Design review of the part built by this model. Coordinates are the model's own, in mm. A direction names the side the tool comes from. Coordinates: 2 decimals unless noted, no trailing zeros. Loops run counter-clockwise (first coordinate to the right, second up) from the corner with the lowest first, then second, coordinate; pieces in that order, holes last. Notation, with made-up numbers: (83.5, 25.25) -> (108.5, 25.25) arc R28 ccw to (108.5, 45.25) -> close; hole circle Ø11 at (61.25, -22.5). An arc over 180 degrees is marked (long way). Answer as a JSON object with one key per item and string values.
Autodesk Inventor part; units mm, degrees
ref_plane "YZ Plane" through (0, 0, 0) normal (1, 0, 0) x (0, 1, 0)
ref_plane "XZ Plane" through (0, 0, 0) normal (0, 1, 0) x (-1, 0, 0)
ref_plane "XY Plane" through (0, 0, 0) normal (0, 0, 1) x (1, 0, 0)
sketch "Szkic1" plane through (0, 0, 0) normal (0, 1, 0) x (-1, 0, 0)
  point P0 (0, 0)
sketch "Szkic2" plane through (0, 0, 0) normal (1, 0, 0) x (0, 1, 0)
  point P0 (0, 0)
sketch "Szkic3" plane through (0, 0, 0) normal (1, 0, 0) x (0, 1, 0)
  line L0 (0, 0) -> (30, 0)
  line L1 (30, 0) -> (30, -36)
  line L2 (30, -36) -> (0, -36)
  line L3 (0, -5) -> (-3, -5)
  line L4 (-3, -5) -> (-3, -31)
  line L5 (-3, -31) -> (0, -31)
  line L6 (0, -36) -> (0, -31)
  line L7 (0, -5) -> (0, 0)
  arc A0 (14.6923, -17.4615) -> (19.3077, -17.4615) centre (17, -23) ccw
  arc A1 (19.3077, -17.4615) -> (14.6923, -17.4615) centre (17, -16.5) ccw
  circle A2 centre (17, -31.5) radius 1.25
  circle A3 centre (17, -4.5) radius 1.25
  dimension "d1" = 36
  dimension "d4" = 5
  dimension "d5" = 26
  dimension "d6" = 3
  dimension "d7" = 30
  dimension "d8" = 13
  dimension "d9" = 13
  dimension "d10" = 4.5
  dimension "d11" = 4.5
  dimension "d12" = 6.5
  dimension "d13" = 12
  dimension "d14" = 5
  dimension "d15" = 2.5
  dimension "d16" = 2.5
extrude "Wyciągnięcie proste1" add sketch "Szkic3" along normal blind 3
properties part number "Podstawa-mocowanie serwa" material "Drewno (wiśnia)"
1) Clearance check with a flat-ended pin moving along its axis: pin 1 Ø11 at (y, z) = (17, -23) entering from +X. State where the tip first meets the part, or that it passes through.
Completed:
{"pin 1": "through"}
2) Add section C-C, the plane x = 0.4. Give the boundary of the cut face in (y, z), and give its area (3 significant figures).
Completed:
{"outline": "(-3, -31) -> (0, -31) -> (0, -36) -> (30, -36) -> (30, 0) -> (0, 0) -> (0, -5) -> (-3, -5) -> close; hole (14.69, -17.46) arc R6 ccw (long way) to (19.31, -17.46) arc R2.5 ccw (long way) to start; hole circle Ø2.5 at (17, -31.5); hole circle Ø2.5 at (17, -4.5)", "area": "1,020 mm²"}
3) For faces 5 (the flat face through (1, -1, -5)), 6 (the flat face through (1, 0, -34)), 7 (the flat face through (1, 30, -18)), list the 3-axis set-ups (+Z, -Z, +X, -X, +Y, -Y) from which the entire face can be reached by the end or side of a thin tool; tool diameter is ignored.
Completed:
{"face 5": "+Z, +X, -X, -Y", "face 6": "-Z, +X, -X, -Y", "face 7": "+Z, -Z, +X, -X, +Y"}
4) Add section B-B, the plane y = 17. Give the boundary of the cut face in (x, z), and give its area (3 significant figures).
Completed:
{"outline": "(0, -36) -> (3, -36) -> (3, -32.75) -> (0, -32.75) -> close; (0, -30.25) -> (3, -30.25) -> (3, -29) -> (0, -29) -> close; (0, -14) -> (3, -14) -> (3, -5.75) -> (0, -5.75) -> close; (0, -3.25) -> (3, -3.25) -> (3, 0) -> (0, 0) -> close", "area": "48.0 mm²"}
5) Add section D-D, the plane z = -23. Give the boundary of the cut face in (x, y).
Completed:
{"outline": "(0, -3) -> (3, -3) -> (3, 11) -> (0, 11) -> close; (0, 23) -> (3, 23) -> (3, 30) -> (0, 30) -> close"}
6) Add section A-A, the plane z = -16.5. Give the boundary of the cut face in (x, y).
Completed:
{"outline": "(0, -3) -> (3, -3) -> (3, 14.5) -> (0, 14.5) -> close; (0, 19.5) -> (3, 19.5) -> (3, 30) -> (0, 30) -> close"}
7) Wall thickness on probe 1 along Z at (x, y) = (2, 17); probe 2 along Y at (x, z) = (1.75, -16.5); probe 3 along Y at (x, z) = (0.95, -23): over which ranges is each line inside the solid? List them lowest first.
Completed:
{"probe 1": "-36 to -32.75, -30.25 to -29, -14 to -5.75, -3.25 to 0", "probe 2": "-3 to 14.5, 19.5 to 30", "probe 3": "-3 to 11, 23 to 30"}
8) The part is to be moulded in two halves that separate along Y. For faces 1 (the cylindrical face through (1.48, 16.73, -3.28)), 2 (the flat face through (1, 0, -3)), 3 (the flat face through (1, 15, 0)), 4 (the cylindrical face through (1, 17, -29)), say which applies: pulls with the +Y half, pulls with the -Y half, needs draft (parallel to the pull), parting line crosses it, or undercut.
Completed:
{"face 1": "undercut", "face 2": "pulls with the -Y half", "face 3": "needs draft", "face 4": "undercut"}
